from build123d import *

# Parameters (mm, degrees)
TABAN_FLAN_1_DEPTH   = 15
M5_DI_LI_DELIK1_D    = 4.2
K_ELERI_START        = -57
K_ELERI_K_R1_DEPTH   = 2
K_ELERI_K_R1_2_DEPTH = 2


# Read off the part's stored shape, not the designer's step: Köşeleri kır1
# Sheet-metal steps are written as plain solids
with BuildPart() as part:
    # Çizim1 → Taban-Flanş1 (new, symmetric)
    with BuildSketch(Plane(origin=(0, 0, 0), x_dir=(0, 0, -1), z_dir=(1, 0, 0))):
        with BuildLine():
            Line((0, 0), (0, -54.2634))
            ThreePointArc((0, -54.2634), (0.215745145, -54.784254855), (0.7366, -55))
            Line((0.7366, -55), (30, -55))
            Line((30, -55), (30, -57))
            Line((30, -57), (0.7366, -57))
            ThreePointArc((0.7366, -57), (-1.198468417, -56.198468417), (-2, -54.2634))
            Line((-2, -54.2634), (-2, 0))
            Line((-2, 0), (0, 0))
        make_face()
    extrude(amount=TABAN_FLAN_1_DEPTH, both=True)

    # M5 Dişli Delik1 (through all)
    with Locations(Plane(origin=(0, -31, 2), x_dir=(1, 0, 0), z_dir=(0, 0, 1))):
        with Locations((0, 0), (0, 25)):
            Hole(M5_DI_LI_DELIK1_D / 2)

    # Köşeleri kır1 outline → Köşeleri kır1 (cut)
    with BuildSketch(Plane(origin=(0, 0, 0), x_dir=(1, 0, 0), z_dir=(0, 1, 0)).offset(K_ELERI_START)):
        with BuildLine():
            Line((15, 30), (10, 30))
            ThreePointArc((10, 30), (13.535533906, 28.535533906), (15, 25))
            Line((15, 25), (15, 30))
        make_face()
        with BuildLine():
            ThreePointArc((-15, 25), (-13.535533906, 28.535533906), (-10, 30))
            Line((-10, 30), (-15, 30))
            Line((-15, 30), (-15, 25))
        make_face()
    extrude(amount=K_ELERI_K_R1_DEPTH, mode=Mode.SUBTRACT)

    # K_eleri k_r1 2 outline → K_eleri k_r1 2 (cut)
    with BuildSketch(Plane.XY):
        with BuildLine():
            Line((-15, 0), (-15, -5))
            ThreePointArc((-15, -5), (-13.535533906, -1.464466094), (-10, 0))
            Line((-10, 0), (-15, 0))
        make_face()
        with BuildLine():
            Line((15, 0), (10, 0))
            ThreePointArc((10, 0), (13.535533906, -1.464466094), (15, -5))
            Line((15, -5), (15, 0))
        make_face()
    extrude(amount=K_ELERI_K_R1_2_DEPTH, mode=Mode.SUBTRACT)


solid = part.part
Check sheet for the modelled part. Datum: model origin and axes. Units: mm. A direction names the side the tool comes from. Round coordinates to 2 decimals unless told otherwise and drop trailing zeros. Write each loop counter-clockwise with the first axis right and the second up, starting at its lowest first coordinate (ties: lowest second). Pieces come first, ordered by that corner, then holes. Notation, with made-up numbers: (62.25, 81.25) - (121.25, 81.25) arc R30 cw to (121.25, 116.25) - close; hole circle Ø7 at (19, 52.5). An arc over 180 degrees is marked (long way). Return JSON: item names as keys, results as strings.
Q1. Draft check along X on faces 3 (the flat face through (0, -28, 2)), 4 (the cylindrical face through (0.46, -33.05, 0.99)), 5 (the cylindrical face through (0.46, -8.05, 0.99)), 6 (the flat face through (-15, -38.6, 0.4)). Enter one of: released by +X, released by -X, zero draft, split by the parting line, or undercut.
Returned:
{"face 3": "zero draft", "face 4": "undercut", "face 5": "undercut", "face 6": "released by -X"}
Q2. Depth check by flat-ended pin: P1, Ø15, axis at x = -7.5, y = -17.5, coming from the -Z side; P2, Ø1.5, axis at x = 7, z = -12, coming from the +Y side. Enter the tip coordinate at first touch or a pass-through.
Returned:
{"P1": "stops at z = 0", "P2": "stops at y = -55"}
Q3. Cross-section at A-A (x = 0). Record the boundary of the cut face in (y, z).
Returned:
{"outline": "(-57, -30) - (-55, -30) - (-55, -0.74) arc R0.74 cw to (-54.26, 0) - (-33.1, 0) - (-33.1, 2) - (-54.26, 2) arc R2.74 ccw to (-57, -0.74) - close; (-28.9, 0) - (-8.1, 0) - (-8.1, 2) - (-28.9, 2) - close; (-3.9, 0) - (0, 0) - (0, 2) - (-3.9, 2) - close"}
Q4. Cross-section at B-B (y = -6). Record the boundary of the cut face in (x, z), then the cut area to 3 significant figures.
Returned:
{"outline": "(-15, 0) - (-2.1, 0) - (-2.1, 2) - (-15, 2) - close; (2.1, 0) - (15, 0) - (15, 2) - (2.1, 2) - close", "area": "51.6 mm²"}
Q5. Scan lines: L1, parallel to Y at x = 3.25, z = -1.5; L2, parallel to Y at x = 0, z = 0.8; L3, parallel to Z at x = 6.75, y = -6. Record each from-to range of solid material in increasing order. Write a range as from..to.
Returned:
{"L1": "y = -57..-55", "L2": "y = -56.53..-33.1, -28.9..-8.1, -3.9..0", "L3": "z = 0..2"}
Q6. Cross-section at D-D (z = -8). Record the boundary of the cut face in (x, y), then the cut area to 3 significant figures.
Returned:
{"outline": "(-15, -57) - (15, -57) - (15, -55) - (-15, -55) - close", "area": "60.0 mm²"}
Q7. Access from +Z, -Z, +X, -X, +Y, -Y to the whole of each face (thin tool, end or side, straight path). Record for faces 1 (the flat face through (0, -55, -15)), 2 (the cylindrical face through (-14, -56, -28)).
Returned:
{"face 1": "-Z, +X, -X, +Y", "face 2": "-Z, -X, +Y, -Y"}
Q8. Cross-section at C-C (x = 4.25). Record the boundary of the cut face in (y, z), then the cut area to 3 significant figures.
Returned:
{"outline": "(-57, -30) - (-55, -30) - (-55, -0.74) arc R0.74 cw to (-54.26, 0) - (0, 0) - (0, 2) - (-54.26, 2) arc R2.74 ccw to (-57, -0.74) - close", "area": "173 mm²"}
